from build123d import *

# Parameters (mm, degrees)
SKETCH1_R           = 3.175
SKETCH1_R_2         = 1.5875
BOSS_EXTRUDE1_DEPTH = 15.875
SKETCH2_R           = 2.032
CUT_EXTRUDE1_DEPTH  = 17.497783942
CIRPATTERN1_COUNT   = 2
CIRPATTERN1_ANGLE   = 90


with BuildPart() as part:
    # Sketch1 → Boss-Extrude1 (new body)
    with BuildSketch(Plane(origin=(0, 0, 0), x_dir=(1, 0, 0), z_dir=(0, 1, 0))):
        with Locations(Location((0, 0, 0), (0, 0, 270))):
            Circle(SKETCH1_R)
        with Locations(Location((0, 0, 0), (0, 0, 270))):
            Circle(SKETCH1_R_2, mode=Mode.SUBTRACT)
    extrude(amount=BOSS_EXTRUDE1_DEPTH)

    # Sketch2 → Cut-Extrude1 (cut, through all)
    with BuildSketch(Plane(origin=(0, 0, 0), x_dir=(0, 0, -1), z_dir=(1, 0, 0))):
        with Locations(Location((0, 5.08, 0), (0, 0, 38.624832873))):
            Circle(SKETCH2_R)
    cut_extrude1 = extrude(amount=-CUT_EXTRUDE1_DEPTH, mode=Mode.SUBTRACT)

    # CirPattern1: Cut-Extrude1 ×2 about axis
    cirpattern1_axis = Axis((0, 0, 0), (0, 1, 0))
    for i in range(1, CIRPATTERN1_COUNT):
        add(cut_extrude1.rotate(cirpattern1_axis, i * CIRPATTERN1_ANGLE / (CIRPATTERN1_COUNT - 1)), mode=Mode.SUBTRACT)


solid = part.part
The model under review builds one solid part; all positions refer to its coordinate system, in mm. A direction names the side the tool comes from. Coordinates: 2 decimals unless noted, no trailing zeros. Write each loop counter-clockwise with the first axis right and the second up, starting at its lowest first coordinate (ties: lowest second). Pieces come first, ordered by that corner, then holes. Notation, with made-up numbers: (84, -13) - (129, -13) arc R27 ccw to (129, 4) - close; hole circle Ø1 at (-9.75, 8). An arc over 180 degrees is marked (long way). Answer as a JSON object with one key per item and string values. Group by question number.
1. Add section B-B (z = 2.5). Give the boundary of the cut face in (x, y) (3 decimals).
2. Clearance check with flat-ended pins moving along their axes: pin 1 Ø1.5 at (x, y) = (1, 3.5) entering from -Z; pin 2 Ø2 at (x, y) = (-2.5, 4) entering from +Z; pin 3 Ø0.5 at (x, y) = (2, 5) entering from +Z; pin 4 Ø3 at (x, z) = (0, 0) entering from +Y. State where each tip first meets the part, or that it passes through.
3. To check wall thickness, follow probe 1 along Y at (x, z) = (-1.25, 2) (3 decimals); probe 2 along Z at (x, y) = (0.75, 10.25); probe 3 along Y at (x, z) = (-2.75, -1) (3 decimals). State the ranges of each line that lie inside material, in increasing order.
4. Mouldability with a two-part tool opening along Z and no side actions: class faces 4 (the face through (2.146, 7.826, -2.34)), 5 (the face through (1.073, 7.826, -1.17)), 6 (the face through (-1.4, 15.875, 1.4)) as pulls with the +Z half, pulls with the -Z half, needs draft (parallel to the pull), parting line crosses it, or undercut.
5. Machinability: for faces 1 (the face through (-1.4, 0, 1.4)), 2 (the face through (2.027, 5.218, 1.918)), 3 (the face through (-1.92, 4.26, -1.86)), which of the approach directions +Z, -Z, +X, -X, +Y, -Y give a long, thin tool a straight path to every point of the face, cutting with its end or side? Answer none if there is none.
6. Add section A-A (x = -2.5). Give the boundary of the cut face in (y, z) (3 decimals), plus the area to 3 significant figures.
7. Add section C-C (z = -0.75). Give the boundary of the cut face in (x, y) (3 decimals).
Findings:
{
 "1": {"outline": "(-1.957, 0) - (1.957, 0) - (1.957, 4.534) arc R2.032 cw to (-1.957, 4.534) - close; (-1.957, 5.626) arc R2.032 cw to (1.957, 5.626) - (1.957, 15.875) - (-1.957, 15.875) - close"},
 "2": {"pin 1": "z = -3.17", "pin 2": "z = 2.78", "pin 3": "z = 2.46", "pin 4": "through"},
 "3": {"probe 1": "0 to 3.478, 6.682 to 15.875", "probe 2": "-3.09 to -1.4, 1.4 to 3.09", "probe 3": "0 to 3.311, 6.849 to 15.875"},
 "4": {"face 4": "parting line crosses it", "face 5": "undercut", "face 6": "needs draft"},
 "5": {"face 1": "+Z, -Z, +X, -X, -Y", "face 2": "+Z", "face 3": "-X"},
 "6": {"outline": "(0, -1.957) - (4.534, -1.957) arc R2.032 cw to (4.534, 1.957) - (0, 1.957) - close; (5.626, -1.957) - (15.875, -1.957) - (15.875, 1.957) - (5.626, 1.957) arc R2.032 cw to start", "area": "49.3 mm²"},
 "7": {"outline": "(-3.085, 0) - (-1.399, 0) - (-1.399, 3.191) - (-3.085, 3.191) - close; (-3.085, 6.969) - (-1.399, 6.969) - (-1.399, 15.875) - (-3.085, 15.875) - close; (1.399, 0) - (3.085, 0) - (3.085, 15.875) - (1.399, 15.875) - close"}
}
